For this review, take the finished solid that the model builds, in its own axes (mm). A direction names the side the tool comes from. Give positions to 0.01 mm unless a question says otherwise; leave off trailing zeros. Write each loop counter-clockwise with the first axis right and the second up, starting at its lowest first coordinate (ties: lowest second). Pieces come first, ordered by that corner, then holes.
1) Draft analysis for pull direction Y (two halves, no side actions). For faces 4 (the face through (304.15, -14.46, 9.22)), 5 (the face through (-1.08, -4.88, -25.94)), 6 (the face through (34, 0, -22)), state which applies: pulls with the +Y half, pulls with the -Y half, needs draft (parallel to the pull), parting line crosses it, or undercut.
2) We need section A-A on x = 35.5. Give the boundary of the cut face in (y, z), and give its area (3 significant figures).
3) For P1, Ø1, axis at y = -10.5, z = 22, coming from the -X side; P2, Ø6, axis at x = 167.5, z = -21, coming from the -Y side; P3, Ø1.5, axis at y = 4, z = -12.5, coming from the +X side; P4, Ø10, axis at y = -6.5, z = -7.5, coming from the -X side, all flat-tipped, find the tip position at first contact; note any pin that passes through.
4) We need section B-B on x = 180.5. Give the boundary of the cut face in (y, z).
5) Machinability: for faces 1 (the face through (318.34, -0.88, -19.98)), 2 (the face through (92, 0, 0)), 3 (the face through (50.744, -4.764, 13.888)), which of the approach directions +Z, -Z, +X, -X, +Y, -Y give a long, thin tool a straight path to every point of the face, cutting with its end or side? Answer none if there is none.
6) Wall thickness on line 1 along Y through (x, z) = (0, -24); line 2 along X through (y, z) = (18, -0.5); line 3 along Z through (x, y) = (72.5, 9): over which ranges is each line inside the solid? List them lowest first.
from build123d import *

# Parameters (mm, degrees)
SALIENTE_EXTRUIR1_DEPTH = 60
CORTAR_EXTRUIR1_REACH   = 135.791
CROQUIS3_W              = 115.000008821
CROQUIS3_H              = 44
CROQUIS6_R              = 6
SALIENTE_EXTRUIR4_DEPTH = 16
CROQUIS7_R              = 4.25
SALIENTE_EXTRUIR5_DEPTH = 12
SALIENTE_EXTRUIR6_REACH = 131.263
CROQUIS8_R              = 6
CROQUIS9_R              = 15.25
SALIENTE_EXTRUIR7_DEPTH = 182
CROQUIS10_R             = 20
SALIENTE_EXTRUIR8_DEPTH = 29
CHAFL_N1_SIZE           = 3
CHAFL_N2_SIZE           = 3
CROQUIS11_R             = 20
SALIENTE_EXTRUIR9_DEPTH = 29
CHAFL_N3_SIZE           = 3
REDONDEO1_R             = 14
CROQUIS12_R             = 5
CORTAR_EXTRUIR2_DEPTH   = 368.658817909


with BuildPart() as part:
    # Croquis1 → Saliente-Extruir1 (new body)
    with BuildSketch(Plane.XY.offset(30)):
        with BuildLine():
            Line((122.000008821, -23), (122.000008821, 23))
            Line((122.000008821, 23), (0, 23))
            ThreePointArc((0, 23), (-23, 0), (0, -23))
            Line((0, -23), (122.000008821, -23))
        make_face()
    extrude(amount=-SALIENTE_EXTRUIR1_DEPTH)

    # Croquis3 → Cortar-Extruir1 (cut, up to next)
    with BuildSketch(Plane(origin=(0, 23, 0), x_dir=(1, 0, 0), z_dir=(0, 1, 0)), mode=Mode.PRIVATE) as cortar_extruir1_sk1:
        with Locations((34.500004411, 0)):
            Rectangle(CROQUIS3_W, CROQUIS3_H)
    cortar_extruir1_tool1 = extrude(cortar_extruir1_sk1.sketch, amount=-CORTAR_EXTRUIR1_REACH, mode=Mode.PRIVATE) & part.part
    add(cortar_extruir1_tool1.solids().sort_by_distance((34.500004, 23, 0))[0], mode=Mode.SUBTRACT)

    # Croquis6 → Saliente-Extruir4 (add)
    with BuildSketch(Plane.XY.offset(-22)):
        with Locations(Location((44.750008821, -4.5, 0), (0, 0, 180))):
            Circle(CROQUIS6_R)
    extrude(amount=SALIENTE_EXTRUIR4_DEPTH)

    # Croquis7 → Saliente-Extruir5 (add)
    with BuildSketch(Plane.XY.offset(-6)):
        with Locations((44.750008821, -4.5)):
            Circle(CROQUIS7_R)
    extrude(amount=SALIENTE_EXTRUIR5_DEPTH)

    # Croquis8 → Saliente-Extruir6 (add, up to next)
    with BuildSketch(Plane.XY.offset(6), mode=Mode.PRIVATE) as saliente_extruir6_sk1:
        with Locations(Location((44.750008821, -4.5, 0), (0, 0, 180))):
            Circle(CROQUIS8_R)
    saliente_extruir6_tool1 = extrude(saliente_extruir6_sk1.sketch, amount=SALIENTE_EXTRUIR6_REACH, mode=Mode.PRIVATE) - part.part
    add(saliente_extruir6_tool1.solids().sort_by_distance((44.750009, -4.5, 6))[0])

    # Croquis9 → Saliente-Extruir7 (add)
    with BuildSketch(Plane(origin=(122.000008821, 0, 0), x_dir=(0, 0, -1), z_dir=(1, 0, 0))):
        Circle(CROQUIS9_R)
    extrude(amount=SALIENTE_EXTRUIR7_DEPTH)

    # Croquis10 → Saliente-Extruir8 (add)
    with BuildSketch(Plane(origin=(304.000008821, 0, 0), x_dir=(0, 0, -1), z_dir=(1, 0, 0))):
        with Locations(Location((0, 0, 0), (0, 0, 180))):
            Circle(CROQUIS10_R)
    extrude(amount=SALIENTE_EXTRUIR8_DEPTH)

    # Chaflán1
    chafl_n1_edges = [part.edges().sort_by_distance(p)[0] for p in [
        (304.000008821, 0, -20),
    ]]
    chamfer(chafl_n1_edges, length=CHAFL_N1_SIZE)

    # Chaflán2
    chafl_n2_edges = [part.edges().sort_by_distance(p)[0] for p in [
        (333.000008821, 0, -20),
    ]]
    chamfer(chafl_n2_edges, length=CHAFL_N2_SIZE)

    # Croquis11 → Saliente-Extruir9 (add)
    with BuildSketch(Plane(origin=(333.000008821, 0, 0), x_dir=(0, 0, -1), z_dir=(1, 0, 0))):
        with Locations(Location((0, 0, 0), (0, 0, 180))):
            Circle(CROQUIS11_R)
    extrude(amount=SALIENTE_EXTRUIR9_DEPTH)

    # Chaflán3
    chafl_n3_edges = [part.edges().sort_by_distance(p)[0] for p in [
        (333.000008821, 0, -20),
    ]]
    chamfer(chafl_n3_edges, length=CHAFL_N3_SIZE - 0.0001)  # a hair under: the kernel refuses the full size

    # Redondeo1
    redondeo1_edges = [part.edges().sort_by_distance(p)[0] for p in [
        (362.000008821, 0, -20),
    ]]
    fillet(redondeo1_edges, radius=REDONDEO1_R)

    # Croquis12 → Cortar-Extruir2 (cut, through all)
    with BuildSketch(Plane.XY.offset(30)):
        Circle(CROQUIS12_R)
    extrude(amount=-CORTAR_EXTRUIR2_DEPTH, mode=Mode.SUBTRACT)


solid = part.part
Results list:
1. face 4: parting line crosses it
1. face 5: undercut
1. face 6: needs draft
2. outline: (-23, -30) - (23, -30) - (23, -22) - (-23, -22) - close; (-23, 22) - (23, 22) - (23, 30) - (-23, 30) - close
2. area: 736 mm2
3. P1: stops at x = -20.71
3. P2: passes through
3. P3: stops at x = 360.46
3. P4: stops at x = 38.75
4. outline: circle Ø30.5 at (0, 0)
5. face 1: +X
5. face 2: +Y, -Y
5. face 3: none
6. line 1: y = -23 to -5, 5 to 23
6. line 2: x = 92 to 122, 305.01 to 331.99, 334.01 to 355.2
6. line 3: z = -30 to -22, 22 to 30
